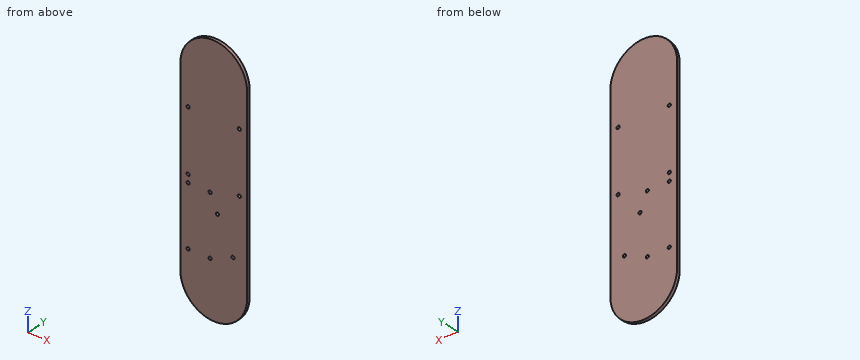
Autodesk Inventor part; units mm, degrees
ref_plane "YZ Plane" through (0, 0, 0) normal (1, 0, 0) x (0, 1, 0)
ref_plane "XZ Plane" through (0, 0, 0) normal (0, 1, 0) x (-1, 0, 0)
ref_plane "XY Plane" through (0, 0, 0) normal (0, 0, 1) x (1, 0, 0)
sketch "Sketch1" plane through (0, 0, 0) normal (0, 1, 0) x (-1, 0, 0)
  line L0 (0, 0) -> (49, 0) construction
  line L1 (49, 0) -> (49, -58) construction
  line L2 (49, -58) -> (0, -58) construction
  line L3 (0, -58) -> (0, 0) construction
  line L4 (53.5, 32) -> (-4.5, 32) construction
  line L5 (-4.5, 32) -> (-4.5, -62) construction
  line L6 (-4.5, -62) -> (53.5, -62) construction
  line L7 (53.5, -62) -> (53.5, 32) construction
  line L8 (53.5, -58) -> (-4.5, -58) construction
  line L9 (24.5, -62) -> (24.5, -133) construction
  line L10 (49, -65.5) -> (28, -65.5) construction
  line L11 (28, -65.5) -> (28, -122.5) construction
  line L12 (28, -122.5) -> (49, -122.5) construction
  line L13 (49, -122.5) -> (49, -65.5) construction
  line L14 (24.5, -94) -> (28, -94) construction
  line L15 (45.5, -122.5) -> (31.5, -122.5) construction
  line L16 (31.5, -122.5) -> (31.5, -140.5) construction
  line L17 (31.5, -140.5) -> (45.5, -140.5) construction
  line L18 (45.5, -140.5) -> (45.5, -122.5) construction
  line L19 (21, -81.75) -> (6, -81.75) construction
  line L20 (6, -81.75) -> (6, -113.25) construction
  line L21 (6, -113.25) -> (21, -113.25) construction
  line L22 (21, -113.25) -> (21, -81.75) construction
  line L23 (24.5, -97.5) -> (21, -97.5) construction
  circle A0 centre (49, -122.5) radius 1.5
  circle A1 centre (49, -65.5) radius 1.5
  circle A2 centre (28, -65.5) radius 1.5
  circle A3 centre (28, -122.5) radius 1.5
  circle A4 centre (49, -58) radius 1.5
  circle A5 centre (0, -58) radius 1.5
  circle A6 centre (0, 0) radius 1.5
  circle A7 centre (49, 0) radius 1.5
  circle A8 centre (21, -81.75) radius 1.5
  circle A9 centre (6, -113.25) radius 1.5
  line L24 (53.5, 32) -> (-4.5, 32) construction
  line L25 (-4.5, 32) -> (-4.5, -140.5) construction
  line L26 (-4.5, -140.5) -> (53.5, -140.5) construction
  line L27 (53.5, -140.5) -> (53.5, 32) construction
  line L28 (56.5, 35) -> (-7.5, 35) construction
  line L29 (-7.5, 35) -> (-7.5, -143.5)
  line L30 (-7.5, -143.5) -> (56.5, -143.5) construction
  line L31 (56.5, -143.5) -> (56.5, 35)
  arc A10 (56.5, 35) -> (-7.5, 35) centre (24.5, 35) ccw
  arc A11 (-7.5, -143.5) -> (56.5, -143.5) centre (24.5, -143.5) ccw
  point P0 (24.5, -58)
  point P1 (38.5, -122.5)
  point P2 (38.5, -140.5)
  point P3 (53.5, -15)
  point P4 (-4.5, -15)
  point P5 (24.5, 32)
  dimension "d0" = 49
  dimension "d1" = 58
  dimension "d2" = 58
  dimension "d3" = 94
  dimension "d4" = 4
  dimension "d7" = 71
  dimension "d8" = 21
  dimension "d9" = 57
  dimension "d10" = 32
  dimension "d11" = 3.5
  dimension "d12" = 14
  dimension "d13" = 18
  dimension "d14" = 15
  dimension "d15" = 31.5
  dimension "d16" = 3.5
  dimension "d17" = 3
  dimension "d18" = 3
  dimension "d19" = 3
  dimension "d20" = 3
  dimension "d21" = 3
  dimension "d22" = 3
  dimension "d23" = 3
  dimension "d24" = 3
  dimension "d25" = 3
  dimension "d26" = 3
  dimension "d27" = 3
extrude "Extrusion1" add sketch "Sketch1" along normal blind 3
properties part number "electronics_layout_v1"
For this review, take the finished solid that the model builds, in its own axes (mm). Round coordinates to 2 decimals unless told otherwise and drop trailing zeros. Loops run counter-clockwise (first coordinate to the right, second up) from the corner with the lowest first, then second, coordinate; pieces in that order, holes last.
Q1. To check wall thickness, follow line 1 along X through (y, z) = (2.3, -65.5); line 2 along Z through (x, y) = (-49, 1.1); line 3 along Z through (x, y) = (0, 2.1). State the ranges of each line that lie inside material, in increasing order.
Result sheet:
line 1: x = -56.5 to -50.5, -47.5 to -29.5, -26.5 to 7.5
line 2: z = -164.09 to -124, -121 to -67, -64 to -59.5, -56.5 to -1.5, 1.5 to 55.59
line 3: z = -164.09 to -59.5, -56.5 to -1.5, 1.5 to 55.59
Q2. Add section B-B on x = -41.5. Write out the cut boundary in (y, z).
Result sheet:
outline: (0, -170.61) - (3, -170.61) - (3, 62.11) - (0, 62.11) - close
Q3. Add section A-A on y = 0.75. Give the number of separate pieces and of enclosed holes in the cut face, plus the area to 3 significant figures.
Result sheet:
separate pieces: 1
enclosed holes: 10
area: 14,600 mm2
